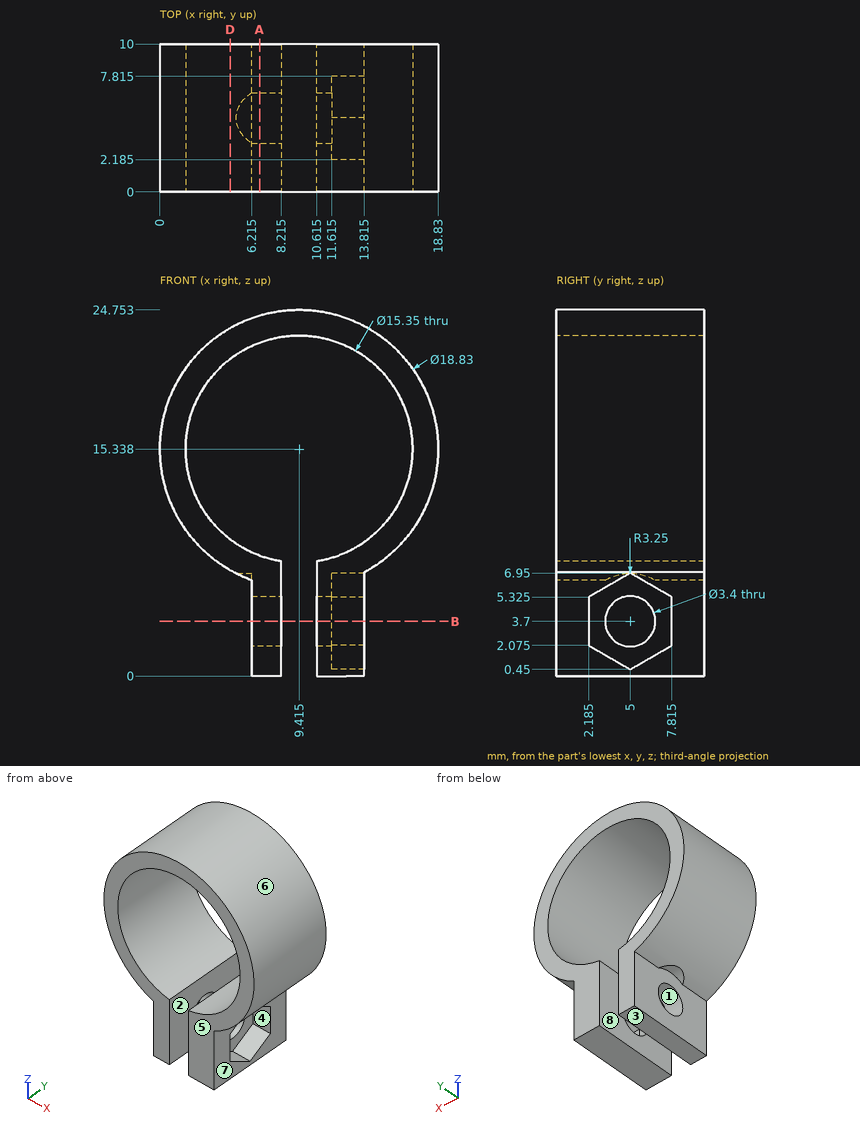
Source: three-view drawing plus pictorial views. Frame: mm from the lowest corner of the part. A direction names the side the tool comes from. Coordinates: 2 decimals unless noted, no trailing zeros. Write each loop counter-clockwise with the first axis right and the second up, starting at its lowest first coordinate (ties: lowest second). Pieces come first, ordered by that corner, then holes. Notation, with made-up numbers: (32, 87.25) -> (81, 87.25) arc R13 cw to (81, 105.25) -> close; hole circle Ø3 at (-39.5, 31.5). An arc over 180 degrees is marked (long way). Write each question's results on one line, items separated by ' | '.
Item 1: Section query B-B on z = 3.7. Return loops of the section in (x, y) (1 decimal).
Conclusion:
outline: (6.2, 0) -> (8.2, 0) -> (8.2, 3.3) -> (6.2, 3.3) -> close; (6.2, 6.7) -> (8.2, 6.7) -> (8.2, 10) -> (6.2, 10) -> close; (10.6, 0) -> (13.8, 0) -> (13.8, 2.2) -> (11.6, 2.2) -> (11.6, 3.3) -> (10.6, 3.3) -> close; (10.6, 6.7) -> (11.6, 6.7) -> (11.6, 7.8) -> (13.8, 7.8) -> (13.8, 10) -> (10.6, 10) -> close
Item 2: Set-up query: the marked faces 4, 5, 6, 7 and 8. Return all of +Z, -Z, +X, -X, +Y, -Y with unobstructed straight access to the full face (end or side cutting, diameter ignored); none if empty.
Conclusion:
face 4: +X | face 5: +Z, -Z, +X, -X, -Y | face 6: +Y, -Y | face 7: -Z, +X, +Y, -Y | face 8: -Z, +Y, -Y
Item 3: Section query D-D on x = 4.75. Return loops of the section in (y, z).
Conclusion:
outline: (0, 7.16) -> (10, 7.16) -> (10, 9.24) -> (0, 9.24) -> close; (0, 21.43) -> (10, 21.43) -> (10, 23.52) -> (0, 23.52) -> close
Item 4: Pin query (flat end, axial travel): pin 1 Ø3.5 at (y, z) = (7, 2.5) entering from +X (3 decimals); pin 2 Ø1 at (y, z) = (2.5, 7.5) entering from -X (1 decimal); pin 3 Ø6 at (y, z) = (7, 5.5) entering from -X (1 decimal). Return the tip coordinate at first contact, or that it passes through.
Conclusion:
pin 1: stops at x = 13.815 | pin 2: stops at x = 3.5 | pin 3: stops at x = 2.9
Item 5: Section query A-A on x = 6.75. Return loops of the section in (y, z) (1 decimal).
Conclusion:
outline: (0, 0) -> (10, 0) -> (10, 8.1) -> (0, 8.1) -> close; (0, 22.5) -> (10, 22.5) -> (10, 24.4) -> (0, 24.4) -> close; hole circle Ø3.4 at (5, 3.7)
Item 6: Mould query, pull axis Z, two halves, no side actions, for the marked faces 1, 2 and 3. Classes: +Z half, -Z half, draft (parallel to the pull), parting line (faces both ways), or undercut.
Conclusion:
face 1: undercut | face 2: draft | face 3: -Z half
Item 7: Material intervals for probe 1 along Y at (x, z) = (7.3, 3.7); probe 2 along X at (y, z) = (3.5, 6) (1 decimal); probe 3 along X at (y, z) = (9, 1.75) (1 decimal), sorted ascending.
Conclusion:
probe 1: y = 0 to 3.3, 6.7 to 10 | probe 2: x = 6.2 to 8.2, 10.6 to 11.6 | probe 3: x = 6.2 to 8.2, 10.6 to 13.8
